```python
from build123d import *

# Parameters (mm, degrees)
SCHIZZO1_W                   = 78.2
SCHIZZO1_H                   = 120
ESTRUSIONE_ESTRUSIONE1_DEPTH = 5
SCHIZZO2_W                   = 78.2
SCHIZZO2_H                   = 120
SCHIZZO2_W_2                 = 74.4
SCHIZZO2_H_2                 = 116.2
ESTRUSIONE_ESTRUSIONE2_DEPTH = 20
SCHIZZO3_W                   = 0.55
SCHIZZO3_H                   = 20
SCHIZZO3_W_2                 = 20
SCHIZZO3_H_2                 = 0.55
ESTRUSIONE_ESTRUSIONE3_DEPTH = 1
SCHIZZO4_W                   = 13
SCHIZZO4_H                   = 13
TAGLIO_ESTRUSIONE1_DEPTH     = 4
RACCORDO1_R                  = 5
RACCORDO2_R                  = 0.5
SCHIZZO5_W                   = 12.2
SCHIZZO5_H                   = 62
TAGLIO_ESTRUSIONE2_DEPTH     = 10


with BuildPart() as part:
    # Schizzo1 → Estrusione-Estrusione1 (new body)
    with BuildSketch(Plane.XY):
        with Locations((0, -18.836070381)):
            Rectangle(SCHIZZO1_W, SCHIZZO1_H)
    extrude(amount=ESTRUSIONE_ESTRUSIONE1_DEPTH)

    # Schizzo2 → Estrusione-Estrusione2 (add)
    with BuildSketch(Plane.XY.offset(5)):
        with Locations((0, -18.836070381)):
            Rectangle(SCHIZZO2_W, SCHIZZO2_H)
        with Locations((0, -18.836070381)):
            Rectangle(SCHIZZO2_W_2, SCHIZZO2_H_2, mode=Mode.SUBTRACT)
    extrude(amount=ESTRUSIONE_ESTRUSIONE2_DEPTH)

    # Schizzo3 → Estrusione-Estrusione3 (add)
    with BuildSketch(Plane.XY.offset(25)):
        with Locations((-38.125, 11.163929619)):
            Rectangle(SCHIZZO3_W, SCHIZZO3_H)
        with Locations((38.127094898, 11.163929619)):
            Rectangle(SCHIZZO3_W, SCHIZZO3_H)
        with Locations((0, 40.188929619)):
            Rectangle(SCHIZZO3_W_2, SCHIZZO3_H_2)
        with Locations((0, -77.861070381)):
            Rectangle(SCHIZZO3_W_2, SCHIZZO3_H_2)
    extrude(amount=ESTRUSIONE_ESTRUSIONE3_DEPTH)

    # Schizzo4 → Taglio-Estrusione1 (cut)
    with BuildSketch(Plane(origin=(39.1, 0, 0), x_dir=(0, 0, -1), z_dir=(1, 0, 0))):
        with Locations((-14.5, 22.663929619)):
            Rectangle(SCHIZZO4_W, SCHIZZO4_H)
    extrude(amount=-TAGLIO_ESTRUSIONE1_DEPTH, mode=Mode.SUBTRACT)

    # Raccordo1
    raccordo1_edges = [part.edges().sort_by_distance(p)[0] for p in [
        (-39.1, 41.163929619, 12.5),
        (39.1, 41.163929619, 12.5),
        (39.1, -78.836070381, 12.5),
        (-39.1, -78.836070381, 12.5),
    ]]
    fillet(raccordo1_edges, radius=RACCORDO1_R)

    # Raccordo2
    raccordo2_edges = [part.edges().sort_by_distance(p)[0] for p in [
        (38.15, 16.163929619, 21),
        (38.15, 29.163929619, 21),
        (38.15, 29.163929619, 8),
        (38.15, 16.163929619, 8),
    ]]
    fillet(raccordo2_edges, radius=RACCORDO2_R)

    # Schizzo5 → Taglio-Estrusione2 (cut)
    with BuildSketch(Plane.ZY.offset(39.1)):
        with Locations((18.9, -47.836070381)):
            Rectangle(SCHIZZO5_W, SCHIZZO5_H)
    extrude(amount=-TAGLIO_ESTRUSIONE2_DEPTH, mode=Mode.SUBTRACT)


solid = part.part
```
Can you work these out from the model? Positions are in its coordinate system, mm. A direction names the side the tool comes from. Coordinates: 2 decimals unless noted, no trailing zeros. Loops run counter-clockwise (first coordinate to the right, second up) from the corner with the lowest first, then second, coordinate; pieces in that order, holes last.
Item 1: Suppose I cut it at A-A (z = 15). Please give me the cut outline in (x, y).
Answers below:
outline: (-39.1, -16.84) - (-37.2, -16.84) - (-37.2, 39.26) - (37.2, 39.26) - (37.2, 29.16) - (39.1, 29.16) - (39.1, 36.16) arc R5 ccw to (34.1, 41.16) - (-34.1, 41.16) arc R5 ccw to (-39.1, 36.16) - close; (-29.1, -78.84) - (34.1, -78.84) arc R5 ccw to (39.1, -73.84) - (39.1, 16.16) - (37.2, 16.16) - (37.2, -76.94) - (-29.1, -76.94) - close
Item 2: Please list where these lines run through material, in increasing order: L1, parallel to X at y = -69, z = 10; L2, parallel to Y at x = -21, z = 23.75; L3, parallel to Z at x = 16.5, y = 5.5.
Answers below:
L1: x = -39.1 to -37.2, 37.2 to 39.1
L2: y = -78.84 to -76.94, 39.26 to 41.16
L3: z = 0 to 5
Item 3: Suppose I cut it at B-B (y = 27). Please give me the cut outline in (x, z), then the cut area to 3 significant figures.
Answers below:
outline: (-39.1, 0) - (39.1, 0) - (39.1, 8) - (37.2, 8) - (37.2, 5) - (-37.2, 5) - (-37.2, 25) - (-39.1, 25) - close; (37.2, 21) - (39.1, 21) - (39.1, 25) - (37.2, 25) - close
area: 442 mm2
Item 4: If we mould it in two halves opening along X, with no side actions, what happens to faces 4 (the face through (-1, -76.936, 15)), 5 (the face through (-37.674, -77.333, 6.49)), 6 (the face through (37.596, 39.738, 12.325))? For each: released by +X, released by -X, zero draft, split by the parting line, or undercut.
Answers below:
face 4: undercut
face 5: released by -X
face 6: released by +X
Item 5: Which directions (+Z, -Z, +X, -X, +Y, -Y) give clear straight access to the entire face, cutting with the end or side of a thin tool? Please do faces 1 (the face through (-38, -50, 12.8)), 2 (the face through (-37.2, -7, 13)), 3 (the face through (0, -78.836, 12)).
Answers below:
face 1: +Z, -X, -Y
face 2: +Z
face 3: +Z, -Z, +X, -X, -Y
Item 6: I'm going to push flat-ended pins straight in: pin 1 (0.6 mm diameter, centred on y = 40, z = 25.5, fed in from -X); pin 2 (1.5 mm diameter, centred on x = 37.5, z = 16, fed in from +Y); pin 3 (2 mm diameter, centred on x = 38, y = 23.5, fed in from +Z). Where does each tip first touch, or does it pass through?
Answers below:
pin 1: stops at x = -10
pin 2: stops at y = 40.4
pin 3: stops at z = 25
Item 7: Suppose I cut it at C-C (x = -3). Please give me the cut outline in (y, z), then the cut area to 3 significant figures.
Answers below:
outline: (-78.84, 0) - (41.16, 0) - (41.16, 25) - (40.46, 25) - (40.46, 26) - (39.91, 26) - (39.91, 25) - (39.26, 25) - (39.26, 5) - (-76.94, 5) - (-76.94, 25) - (-77.59, 25) - (-77.59, 26) - (-78.14, 26) - (-78.14, 25) - (-78.84, 25) - close
area: 677 mm2
Item 8: Suppose I cut it at D-D (y = -52.5). Please give me the cut outline in (x, z).
Answers below:
outline: (-39.1, 0) - (39.1, 0) - (39.1, 25) - (37.2, 25) - (37.2, 5) - (-37.2, 5) - (-37.2, 12.8) - (-39.1, 12.8) - close
